Design review of the part built by this model. Coordinates are the model's own, in mm. Round coordinates to 2 decimals unless told otherwise and drop trailing zeros. Order: outer loops, then holes, each group sorted by start corner. A loop starts at its lowest first (then second) coordinate and runs counter-clockwise, first axis right, second up. Notation, with made-up numbers: M -35,-13.5 L -12,-13.5 A25 cw -12,13.5 Z; hole C -19.75,-29 d2. An arc over 180 degrees is marked long. Write item = value, one per line. Start each with the question number.
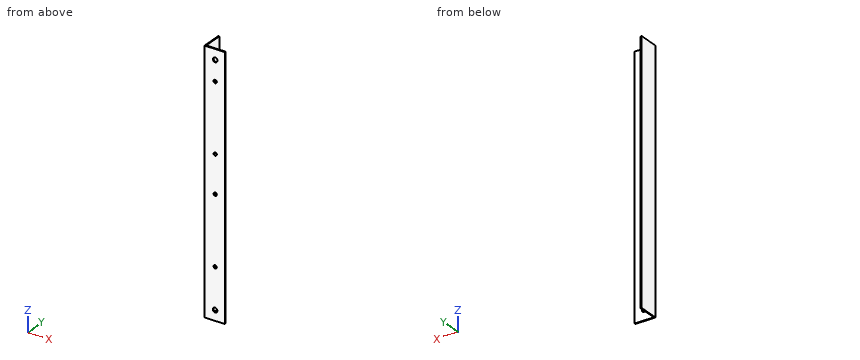
```python
from build123d import *

# Parameters (mm, degrees)
EXTRUDE_1_DEPTH     = 251
SKETCH_2_R          = 1.6
CUT_EXTRUDE_1_DEPTH = 2
SKETCH_3_R          = 2.25
CUT_EXTRUDE_2_DEPTH = 2


with BuildPart() as part:
    # Эскиз1 → Бобышка-Вытянуть1 (new body)
    with BuildSketch(Plane.XY):
        Polygon((0, 0), (0, 20), (1, 20), (1, 1), (20, 1), (20, 0), align=None)
    extrude(amount=EXTRUDE_1_DEPTH)

    # Эскиз2 → Вырез-Вытянуть1 (cut, through all)
    with BuildSketch(Plane(origin=(0, 1, 0), x_dir=(1, 0, 0), z_dir=(0, 1, 0))):
        with Locations((10.5, -50)):
            Circle(SKETCH_2_R)
        with Locations((10.5, -117)):
            Circle(SKETCH_2_R)
        with Locations((10.5, -221)):
            Circle(SKETCH_2_R)
        with Locations((10.5, -154)):
            Circle(SKETCH_2_R)
    extrude(amount=-CUT_EXTRUDE_1_DEPTH, mode=Mode.SUBTRACT)

    # Эскиз3 → Вырез-Вытянуть2 (cut, through all)
    with BuildSketch(Plane(origin=(0, 1, 0), x_dir=(1, 0, 0), z_dir=(0, 1, 0))):
        with Locations((10.5, -241)):
            Circle(SKETCH_3_R)
        with Locations((10.5, -10)):
            Circle(SKETCH_3_R)
    extrude(amount=-CUT_EXTRUDE_2_DEPTH, mode=Mode.SUBTRACT)


solid = part.part
```
(1) Consider section A-A, the plane z = 10. Write out the cut boundary in (x, y).
(2) Insertion check: pin 1 (1 mm diameter, centred on x = 8.5, z = 104.5, fed in from +Y); pin 2 (1.5 mm diameter, centred on y = 17.5, z = 165, fed in from +X). Each pin has a flat end and moves straight along its axis. Give the tip position at first contact, or say it passes through.
(3) Consider section B-B, the plane x = 3.75. Write out the cut boundary in (y, z).
(4) For line 1 along X through (y, z) = (0.75, 117); line 2 along X through (y, z) = (0.75, 10); line 3 along Y through (x, z) = (3.25, 199), list the stretches that pass through material, from the lowest coordinate up. Write a range as [from, to].
Completed:
q1.outline = M 0,0 L 8.25,0 L 8.25,1 L 1,1 L 1,20 L 0,20 Z; M 12.75,0 L 20,0 L 20,1 L 12.75,1 Z
q2.pin_1 = 1
q2.pin_2 = 1
q3.outline = M 0,0 L 1,0 L 1,251 L 0,251 Z
q4.line_1 = [0, 8.9], [12.1, 20]
q4.line_2 = [0, 8.25], [12.75, 20]
q4.line_3 = [0, 1]
